Work out the finished part from the listing and answer in its coordinate system (mm). Round coordinates to 2 decimals unless told otherwise and drop trailing zeros. Order: outer loops, then holes, each group sorted by start corner. A loop starts at its lowest first (then second) coordinate and runs counter-clockwise, first axis right, second up. Notation, with made-up numbers: (1.5, 34.5) - (48.5, 34.5) arc R23 cw to (48.5, 48.5) - close; hole circle Ø10 at (28, -23). An arc over 180 degrees is marked (long way). Put each result on its own line as item: value.
```python
from build123d import *

# Parameters (mm, degrees)
SKETCH1_W               = 525.399648274
SKETCH1_H               = 377.876053004
BOSS_EXTRUDE1_DEPTH     = 6
CUT_EXTRUDE_THIN2_DEPTH = 324.642975299


with BuildPart() as part:
    # Sketch1 → Boss-Extrude1 (new body)
    with BuildSketch(Plane(origin=(0, 0, 0), x_dir=(1, 0, 0), z_dir=(0, 1, 0))):
        Rectangle(SKETCH1_W, SKETCH1_H)
    extrude(amount=BOSS_EXTRUDE1_DEPTH)

    # Sketch2 → Cut-Extrude-Thin2 (cut, through all)
    with BuildSketch(Plane(origin=(0, 6, 0), x_dir=(1, 0, 0), z_dir=(0, 1, 0))):
        Polygon((-187.350784755, 75.591944913), (-187.350784755, 51.841944259), (-187.411415821, 51.841944259), (-187.411415821, 11.331943142), (-187.350784755, 11.331943142), (-187.350784755, -12.418057512), (-129.745802698, -12.418057512), (-129.745802698, -18.418057678), (-89.235801582, -18.418057678), (-89.235801582, -12.418057512), (-48.745800465, -12.418057512), (-48.745800465, -18.418057678), (-8.235799349, -18.418057678), (-8.235799349, -12.418057512), (32.254201767, -12.418057512), (32.254201767, -18.418057678), (72.764202884, -18.418057678), (72.764202884, -12.418057512), (113.254204, -12.418057512), (113.254204, -18.418057678), (153.764205117, -18.418057678), (153.764205117, -12.418057512), (194.259206233, -12.418057512), (211.369187173, -12.418057512), (211.369187173, 11.336943142), (211.369187173, 51.836944259), (211.369187173, 75.591944913), (153.764205117, 75.591944913), (153.764205117, 81.591945079), (113.254204, 81.591945079), (113.254204, 75.591944913), (72.764202884, 75.591944913), (72.764202884, 81.591945079), (32.254201767, 81.591945079), (32.254201767, 75.591944913), (-8.235799349, 75.591944913), (-8.235799349, 81.591945079), (-48.745800465, 81.591945079), (-48.745800465, 75.591944913), (-89.235801582, 75.591944913), (-89.235801582, 81.591945079), (-129.745802698, 81.591945079), (-129.745802698, 75.591944913), (-170.240803815, 75.591944913), align=None)
        Polygon((-187.340784755, 75.581944913), (-187.340784755, 51.831944259), (-187.401415821, 51.831944259), (-187.401415821, 11.341943142), (-187.340784755, 11.341943142), (-187.340784755, -12.408057512), (-129.735802698, -12.408057512), (-129.735802698, -18.408057678), (-89.245801582, -18.408057678), (-89.245801582, -12.408057512), (-48.735800465, -12.408057512), (-48.735800465, -18.408057678), (-8.245799349, -18.408057678), (-8.245799349, -12.408057512), (32.264201767, -12.408057512), (32.264201767, -18.408057678), (72.754202884, -18.408057678), (72.754202884, -12.408057512), (113.264204, -12.408057512), (113.264204, -18.408057678), (153.754205117, -18.408057678), (153.754205117, -12.408057512), (194.259206233, -12.408057512), (211.359187173, -12.408057512), (211.359187173, 11.336943142), (211.359187173, 51.836944259), (211.359187173, 75.581944913), (153.754205117, 75.581944913), (153.754205117, 81.581945079), (113.264204, 81.581945079), (113.264204, 75.581944913), (72.754202884, 75.581944913), (72.754202884, 81.581945079), (32.264201767, 81.581945079), (32.264201767, 75.581944913), (-8.245799349, 75.581944913), (-8.245799349, 81.581945079), (-48.735800465, 81.581945079), (-48.735800465, 75.581944913), (-89.245801582, 75.581944913), (-89.245801582, 81.581945079), (-129.735802698, 81.581945079), (-129.735802698, 75.581944913), (-170.240803815, 75.581944913), align=None, mode=Mode.SUBTRACT)
    extrude(amount=-CUT_EXTRUDE_THIN2_DEPTH, mode=Mode.SUBTRACT)


with BuildPart() as body_2:
    # of the pieces the cut leaves, the one that is kept (cut_extrude_thin2_keep)
    add(part.part.solids().sort_by_distance((-129.735802698, 0, -75.581944913))[0])


solid = body_2.part
```
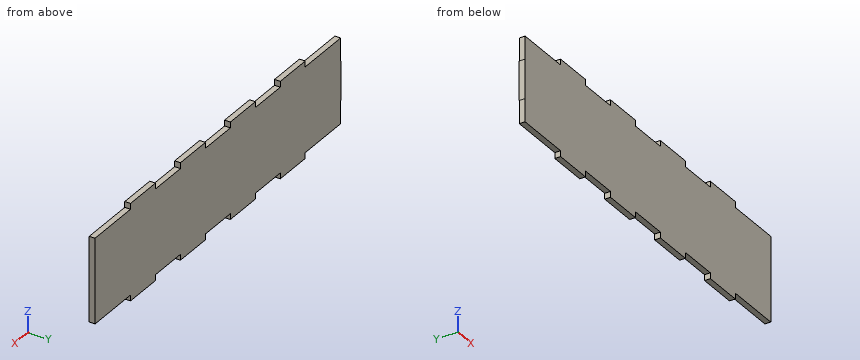
1) Straight lines are drawn through the part: L1, parallel to X at y = 1.9, z = -75; L2, parallel to Z at x = -148, y = 4.45. For each, find the intervals that lie inside material, in ascending order. Write a range as from..to.
Findings below:
L1: x = -187.34..211.36
L2: z = -75.58..12.41
2) Given pin 1 Ø1.8 at (y, z) = (4.5, -79.5) entering from +X; pin 2 Ø1.8 at (y, z) = (2, -79) entering from -X; pin 3 Ø1.8 at (x, y) = (-168.5, 1.5) entering from +Z; pin 4 Ø1.5 at (x, z) = (-131.5, -69) entering from -Y, each flat-ended and moving along its own axis, determine where each tip first touches the part or whether it passes through.
Findings below:
pin 1: stops at x = 153.75
pin 2: stops at x = -129.74
pin 3: stops at z = 12.41
pin 4: stops at y = 0
3) A cutting plane is placed at A-A on x = 16. Write down the section's boundary in (y, z).
Findings below:
outline: (0, -75.58) - (6, -75.58) - (6, 12.41) - (0, 12.41) - close
